from build123d import *

# Parameters (mm, degrees)
SKETCH1_W           = 25.4
SKETCH1_H           = 114.3
BOSS_EXTRUDE1_DEPTH = 6.35
SKETCH2_R           = 5.5626
BOSS_EXTRUDE2_DEPTH = 3.175
SKETCH3_R           = 5.5626
BOSS_EXTRUDE3_DEPTH = 1.799999956
BOSS_EXTRUDE4_REACH = 119.26
CUT_EXTRUDE1_START  = -4.974999956
CUT_EXTRUDE1_DEPTH  = 4.974999956
FILLET1_R           = 0.508


with BuildPart() as part:
    # Sketch1 → Boss-Extrude1 (new body)
    with BuildSketch(Plane.XY):
        with Locations((12.7, 57.15)):
            Rectangle(SKETCH1_W, SKETCH1_H)
    extrude(amount=-BOSS_EXTRUDE1_DEPTH)

    # Sketch2 → Boss-Extrude2 (add)
    with BuildSketch(Plane.XY):
        with Locations(Location((12.7, 107.5182, 0), (0, 0, 180))):
            Circle(SKETCH2_R)
    extrude(amount=BOSS_EXTRUDE2_DEPTH)

    # Sketch3 → Boss-Extrude3 (add)
    with BuildSketch(Plane.XY.offset(3.175)):
        with Locations(Location((12.7, 104.9782, 0), (0, 0, 166.802375663))):
            Circle(SKETCH3_R)
    extrude(amount=BOSS_EXTRUDE3_DEPTH)

    # Boss-Extrude4: up to this face of the body (flat: up to its plane)
    boss_extrude4_end = Plane(part.part.faces().sort_by_distance((12.7, 104.9782, 4.974999956))[0])
    # Sketch4 → Boss-Extrude4 (add, up to the picked face)
    with BuildSketch(Plane.XY, mode=Mode.PRIVATE) as boss_extrude4_sk1:
        with BuildLine():
            Line((14.732, 107.5182), (14.732, 90.2208))
            ThreePointArc((14.732, 90.2208), (12.7, 88.1888), (10.668, 90.2208))
            Line((10.668, 90.2208), (10.668, 107.5182))
            ThreePointArc((10.668, 107.5182), (12.7, 109.5502), (14.732, 107.5182))
        make_face()
    boss_extrude4_tool1 = split(extrude(boss_extrude4_sk1.sketch, amount=BOSS_EXTRUDE4_REACH, mode=Mode.PRIVATE), bisect_by=boss_extrude4_end, keep=Keep.BOTH, mode=Mode.PRIVATE)
    add(boss_extrude4_tool1.solids().sort_by(Axis((12.7, 98.8695, 0), (0, 0, 1)))[0])

    # Sketch5 → Cut-Extrude1 (cut)
    with BuildSketch(Plane.XY.offset(4.974999956).offset(CUT_EXTRUDE1_START)):
        with BuildLine():
            Line((7.1374, 114.3), (7.1374, 104.9782))
            ThreePointArc((7.1374, 104.9782), (12.7, 110.5408), (18.2626, 104.9782))
            Line((18.2626, 104.9782), (18.2626, 114.3))
            Line((18.2626, 114.3), (7.1374, 114.3))
        make_face()
    extrude(amount=CUT_EXTRUDE1_DEPTH, mode=Mode.SUBTRACT)

    # Fillet1
    fillet1_edges = [part.edges().sort_by_distance(p)[0] for p in [
        (10.668, 102.340025152, 1.5875),
        (10.668, 99.800025152, 4.074999978),
        (14.732, 102.340025152, 1.5875),
        (14.732, 99.800025152, 4.074999978),
    ]]
    fillet(fillet1_edges, radius=FILLET1_R)


solid = part.part
For this review, take the finished solid that the model builds, in its own axes (mm). A direction names the side the tool comes from. Round coordinates to 2 decimals unless told otherwise and drop trailing zeros. Write each loop counter-clockwise with the first axis right and the second up, starting at its lowest first coordinate (ties: lowest second). Pieces come first, ordered by that corner, then holes. Notation, with made-up numbers: M 83.25,44 L 95.25,44 A4 ccw 95.25,50 Z; hole C -12,56.25 d4. An arc over 180 degrees is marked long. Write item = value, one per line. Start each with the question number.
(1) We need section A-A (x = 12.7). Give the boundary of the cut face in (y, z) (3 decimals).
(2) Clearance check with a flat-ended pin moving along its axis: pin 1 Ø12.5 at (x, y) = (11.5, 39) entering from +Z. State where the tip first meets the part, or that it passes through.
(3) For line 1 along Z through (x, y) = (22.25, 49.5); line 2 along X through (y, z) = (94, 4.25); line 3 along Y through (x, z) = (11.25, 3.5), list the stretches that pass through material, from the lowest coordinate up.
(4) For faces 1 (the face through (13, 0, -3)), 2 (the face through (25.4, 56, -3)), 3 (the face through (8.369, 104.028, 1.565)), 4 (the face through (16.986, 103.973, 1.565)), 5 (the face through (12.911, 110.537, 3.005)), list the 3-axis set-ups (+Z, -Z, +X, -X, +Y, -Y) from which the entire face can be reached by the end or side of a thin tool; tool diameter is ignored.
(5) We need section B-B (y = 71). Give the boundary of the cut face in (x, z), then the cut area to 3 significant figures.
(6) The part is to be moulded in two halves that separate along Z. For faces 6 (the face through (9, 102, 3.175)), 7 (the face through (12.74, 88.19, 2.45)), 8 (the face through (13, 58, -6.35)), say which applies: +Z half, -Z half, draft (parallel to the pull), parting line (faces both ways), or undercut.
Results found:
q1.outline = M 0,-6.35 L 114.3,-6.35 L 114.3,0 L 110.541,0 L 110.541,4.975 L 88.189,4.975 L 88.189,0 L 0,0 Z
q2.pin_1 = 0
q3.line_1 = -6.35 to 0
q3.line_2 = 10.67 to 14.73
q3.line_3 = 88.8 to 110.35
q4.face_1 = +Z, -Z, +X, -X, -Y
q4.face_2 = +Z, -Z, +X, +Y, -Y
q4.face_3 = -X, -Y
q4.face_4 = +X, -Y
q4.face_5 = +Z
q5.outline = M 0,-6.35 L 25.4,-6.35 L 25.4,0 L 0,0 Z
q5.area = 161 mm²
q6.face_6 = undercut
q6.face_7 = draft
q6.face_8 = -Z half
